Input: dimensioned drawing with shaded views. Units: mm. Origin: part minimum x, y, z. Round coordinates to 2 decimals unless told otherwise and drop trailing zeros. Loops run counter-clockwise (first coordinate to the right, second up) from the corner with the lowest first, then second, coordinate; pieces in that order, holes last.
Item 1: Section query B-B on x = 17. Return loops of the section in (y, z), then the cut area to 3 significant figures.
Item 2: Ray query, L1, parallel to X at y = 0.5, z = 11.5; L2, parallel to Z at x = 3.25, y = 0.9; L3, parallel to Z at x = 11.75, y = 0.7. Return the intervals inside material, ascending.
Item 3: Section query A-A on y = 0.3. Return loops of the section in (x, z), then the cut area to 3 significant figures.
Item 4: First-contact query: P1, Ø0.5, axis at y = 0.5, z = 19, coming from the -X side. Flat tip, straight axial feed; report the tip coordinate or a pass-through.
Item 5: Section query C-C on z = 28.5. Return loops of the section in (x, y), then the cut area to 3 significant figures.
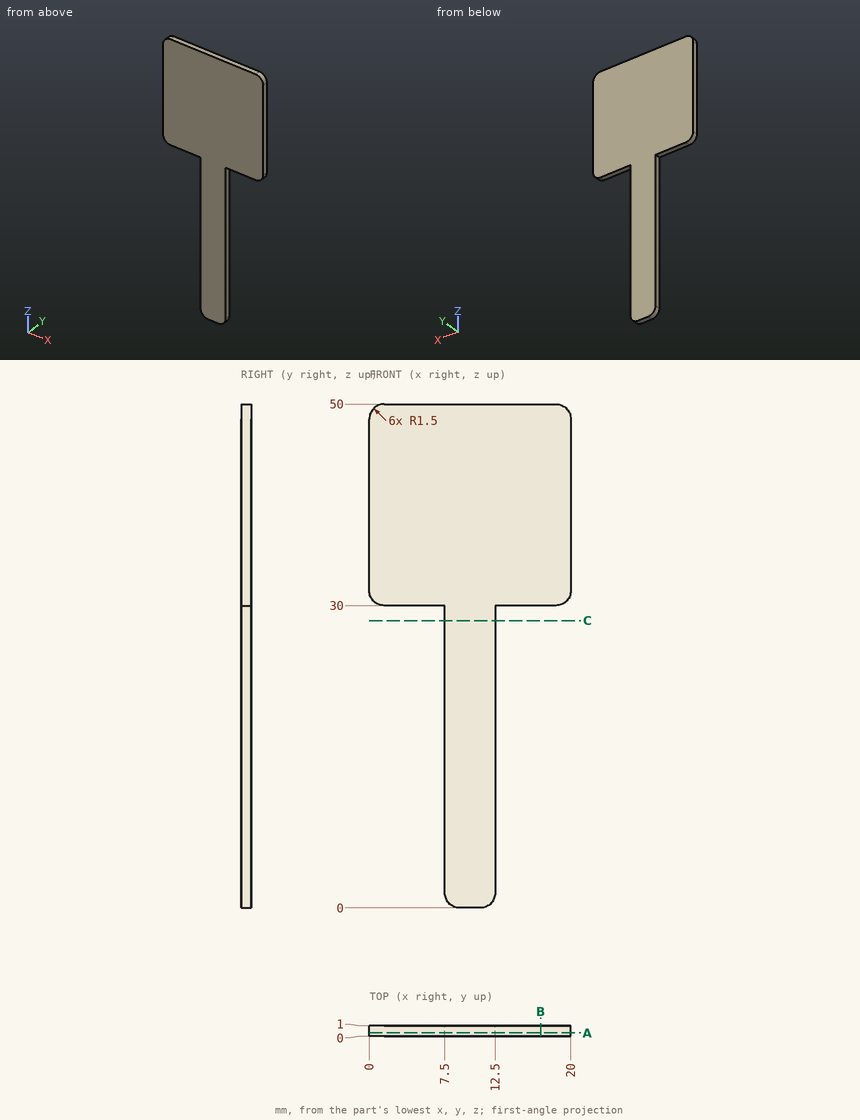
Data:
1. outline: (0, 30) - (1, 30) - (1, 50) - (0, 50) - close
1. area: 20.0 mm2
2. L1: x = 7.5 to 12.5
2. L2: z = 30 to 50
2. L3: z = 0.2 to 50
3. outline: (0, 31.5) arc R1.5 ccw to (1.5, 30) - (7.5, 30) - (7.5, 1.5) arc R1.5 ccw to (9, 0) - (11, 0) arc R1.5 ccw to (12.5, 1.5) - (12.5, 30) - (18.5, 30) arc R1.5 ccw to (20, 31.5) - (20, 48.5) arc R1.5 ccw to (18.5, 50) - (1.5, 50) arc R1.5 ccw to (0, 48.5) - close
3. area: 547 mm2
4. P1: stops at x = 7.5
5. outline: (7.5, 0) - (12.5, 0) - (12.5, 1) - (7.5, 1) - close
5. area: 5.00 mm2
